Check sheet for the modelled part. Datum: model origin and axes. Units: mm. Face numbers are marked on the shaded views. A direction names the side the tool comes from. Round coordinates to 2 decimals unless told otherwise and drop trailing zeros. Loops run counter-clockwise (first coordinate to the right, second up) from the corner with the lowest first, then second, coordinate; pieces in that order, holes last. Notation, with made-up numbers: (-2, 77) -> (25, 77) arc R29 ccw to (25, 116) -> close; hole circle Ø11 at (-31, -37.75). An arc over 180 degrees is marked (long way). One line per item, written item: value. Start each with the question number.
1. Go/stop test with flat-tipped pins: pin 1 (5 mm diameter, centred on x = 119.5, y = 32, fed in from -Z); pin 2 (1 mm diameter, centred on y = 42.5, z = -11, fed in from -X); pin 3 (3 mm diameter, centred on x = 88, y = 40, fed in from +Z). Record where each tip stops, or that it passes through.
2. Cross-section at C-C on y = 70. Record the cut outline in (x, z).
3. Cross-section at D-D on x = 211.5. Record the cut outline in (y, z).
4. Set-up check for the marked faces 5, 6 and 7: record each of +Z, -Z, +X, -X, +Y, -Y from which the full face is reachable in a straight line by a thin tool's end or side.
5. Cross-section at A-A on x = 20. Record the cut outline in (y, z).
6. Cross-section at B-B on z = 13. Record the cut outline in (x, y), then the cut area to 3 significant figures.
7. Release check for a two-part mould opening along X. For the marked faces 1, 2, 3 and 4 record: +X half, -X half, draft (parallel to the pull), parting line (faces both ways), or undercut.
8. Material ranges on L1, parallel to X at y = 85.95, z = 13; L2, parallel to Z at x = 245, y = 86.55; L3, parallel to Y at x = 152.5, z = 18.5, recorded low to high.
from build123d import *

# Parameters (mm, degrees)
SKETCH1_W           = 265
SKETCH1_H           = 85
BOSS_EXTRUDE2_DEPTH = 25
SHELL1_T            = 2
SKETCH3_W           = 50
SKETCH3_H           = 20
BOSS_EXTRUDE3_DEPTH = 1
SKETCH5_R           = 2.5
CUT_EXTRUDE1_DEPTH  = 87


with BuildPart() as part:
    # Sketch1 → Boss-Extrude2 (new body)
    with BuildSketch(Plane.XY):
        with Locations((132.5, 42.5)):
            Rectangle(SKETCH1_W, SKETCH1_H)
    extrude(amount=BOSS_EXTRUDE2_DEPTH)

    # Shell1
    shell1_openings = [part.faces().sort_by_distance(p)[0] for p in [
        (132.5, 42.5, 25),
    ]]
    offset(amount=SHELL1_T, openings=shell1_openings, kind=Kind.INTERSECTION)

    # Sketch3 → Boss-Extrude3 (add, symmetric)
    with BuildSketch(Plane(origin=(0, 42.5, 0), x_dir=(1, 0, 0), z_dir=(0, 1, 0))):
        with Locations((132.5, 12)):
            Rectangle(SKETCH3_W, SKETCH3_H)
    extrude(amount=BOSS_EXTRUDE3_DEPTH, both=True)

    # Sketch5 → Cut-Extrude1 (cut)
    with BuildSketch(Plane(origin=(0, 87, 0), x_dir=(1, 0, 0), z_dir=(0, 1, 0))):
        with Locations(Location((245, -13, 0), (0, 0, 270))):
            Circle(SKETCH5_R)
        with Locations(Location((20, -13, 0), (0, 0, 270))):
            Circle(SKETCH5_R)
    cut_extrude1 = extrude(amount=-CUT_EXTRUDE1_DEPTH, mode=Mode.SUBTRACT)

    # Mirror1: Cut-Extrude1 across plane
    add(cut_extrude1.mirror(Plane.ZX.offset(42.5)), mode=Mode.SUBTRACT)


solid = part.part
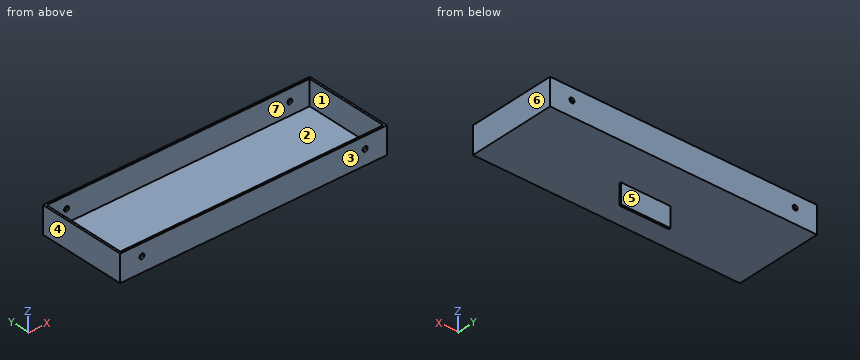
Taken from the geometry:
1. pin 1: stops at z = -2
1. pin 2: stops at x = 107.5
1. pin 3: stops at z = 0
2. outline: (-2, -2) -> (267, -2) -> (267, 25) -> (265, 25) -> (265, 0) -> (0, 0) -> (0, 25) -> (-2, 25) -> close
3. outline: (-2, -2) -> (87, -2) -> (87, 25) -> (85, 25) -> (85, 0) -> (0, 0) -> (0, 25) -> (-2, 25) -> close
4. face 5: -Z, +X, -X, +Y
4. face 6: +Z, -Z, +X, +Y, -Y
4. face 7: +Z
5. outline: (-2, -2) -> (87, -2) -> (87, 10.5) -> (85, 10.5) -> (85, 0) -> (0, 0) -> (0, 10.5) -> (-2, 10.5) -> close; (-2, 15.5) -> (0, 15.5) -> (0, 25) -> (-2, 25) -> close; (85, 15.5) -> (87, 15.5) -> (87, 25) -> (85, 25) -> close
6. outline: (-2, -2) -> (17.5, -2) -> (17.5, 0) -> (0, 0) -> (0, 85) -> (17.5, 85) -> (17.5, 87) -> (-2, 87) -> close; (22.5, -2) -> (242.5, -2) -> (242.5, 0) -> (22.5, 0) -> close; (22.5, 85) -> (242.5, 85) -> (242.5, 87) -> (22.5, 87) -> close; (247.5, -2) -> (267, -2) -> (267, 87) -> (247.5, 87) -> (247.5, 85) -> (265, 85) -> (265, 0) -> (247.5, 0) -> close
6. area: 1,380 mm2
7. face 1: undercut
7. face 2: undercut
7. face 3: draft
7. face 4: -X half
8. L1: x = -2 to 17.5, 22.5 to 242.5, 247.5 to 267
8. L2: z = -2 to 10.5, 15.5 to 25
8. L3: y = -2 to 0, 85 to 87
